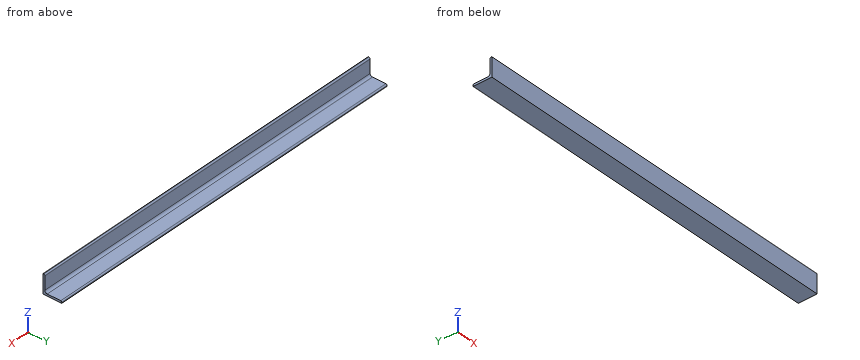
```python
from build123d import *

# Parameters (mm, degrees)
F1_DEPTH = 800


with BuildPart() as f1:
    # F0 (on Right) → F1 (new body, symmetric)
    with BuildSketch(Plane.YZ):
        with BuildLine():
            Line((0, 0), (80, 0))
            Line((80, 0), (80, 3))
            ThreePointArc((80, 3), (78.535534, 6.535534), (75, 8))
            Line((75, 8), (18, 8))
            ThreePointArc((18, 8), (10.928932, 10.928932), (8, 18))
            Line((8, 18), (8, 75))
            ThreePointArc((8, 75), (6.535534, 78.535534), (3, 80))
            Line((3, 80), (0, 80))
            Line((0, 80), (0, 0))
        make_face()
    extrude(amount=F1_DEPTH, both=True)


solid = f1.part
```
Input: part model. Units: mm. Frame: model coordinates. Round coordinates to 2 decimals unless told otherwise and drop trailing zeros. Loops run counter-clockwise (first coordinate to the right, second up) from the corner with the lowest first, then second, coordinate; pieces in that order, holes last. Notation, with made-up numbers: (-18.5, -17) -> (8.5, -17) arc R22 ccw to (8.5, -4) -> close; hole circle Ø9 at (21, 35). An arc over 180 degrees is marked (long way). Use one line per item in the form item = value. Start each with the question number.
Item 1: Contact query for flat-ended pins moving along their axis: pin 1 Ø4 at (x, z) = (-291, 66) entering from +Y; pin 2 Ø1.5 at (x, y) = (28.5, 39.5) entering from +Z. Output: stop coordinate, or through.
Item 2: Section query A-A on x = -77. Return the cut outline in (y, z), then the cut area to 3 significant figures.
Item 3: Material intervals for L1, parallel to Z at x = 236.5, y = 32; L2, parallel to Z at x = -612.5, y = 16, sorted ascending. Write a range as from..to.
Item 4: Section query B-B on z = 31. Return the cut outline in (x, y), then the cut area to 3 significant figures.
Ans:
q1.pin_1 = 8
q1.pin_2 = 8
q2.outline = (0, 0) -> (80, 0) -> (80, 3) arc R5 ccw to (75, 8) -> (18, 8) arc R10 cw to (8, 18) -> (8, 75) arc R5 ccw to (3, 80) -> (0, 80) -> close
q2.area = 1,230 mm^2
q3.L1 = 0..8
q3.L2 = 0..8.2
q4.outline = (-800, 0) -> (800, 0) -> (800, 8) -> (-800, 8) -> close
q4.area = 12,800 mm^2
